from build123d import *

# Parameters (mm, degrees)
SKETCH1_R           = 17.5
SKETCH1_R_2         = 10
SKETCH1_R_3         = 2
BOSS_EXTRUDE1_DEPTH = 3.5
SKETCH3_R           = 10.5
BOSS_EXTRUDE2_DEPTH = 14
FILLET1_R           = 4
SKETCH4_R           = 6
BOSS_EXTRUDE3_DEPTH = 5
FILLET2_R           = 5


with BuildPart() as part:
    # Sketch1 → Boss-Extrude1 (new body)
    with BuildSketch(Plane.XY):
        Circle(SKETCH1_R)
        Circle(SKETCH1_R_2, mode=Mode.SUBTRACT)
        with Locations((6.70392983, 12.290538021)):
            Circle(SKETCH1_R_3, mode=Mode.SUBTRACT)
        with Locations((7.291953237, -11.951042548)):
            Circle(SKETCH1_R_3, mode=Mode.SUBTRACT)
        with Locations((-13.995883067, -0.339495473)):
            Circle(SKETCH1_R_3, mode=Mode.SUBTRACT)
    extrude(amount=BOSS_EXTRUDE1_DEPTH)

    # Sketch3 → Boss-Extrude2 (add)
    with BuildSketch(Plane.XY.offset(3.5)):
        Circle(SKETCH3_R)
    extrude(amount=BOSS_EXTRUDE2_DEPTH)

    # Fillet1
    fillet1_edges = [part.edges().sort_by_distance(p)[0] for p in [
        (-10.5, 0, 17.5),
    ]]
    fillet(fillet1_edges, radius=FILLET1_R)

    # Sketch4 → Boss-Extrude3 (add)
    with BuildSketch(Plane.XY.offset(17.5)):
        Circle(SKETCH4_R)
    extrude(amount=BOSS_EXTRUDE3_DEPTH)

    # Fillet2
    fillet2_edges = [part.edges().sort_by_distance(p)[0] for p in [
        (-6, 0, 22.5),
    ]]
    fillet(fillet2_edges, radius=FILLET2_R - 0.0001)  # a hair under: the kernel refuses the full size


solid = part.part
Work out the finished part from the listing and answer in its coordinate system (mm). A direction names the side the tool comes from. Coordinates: 2 decimals unless noted, no trailing zeros. Write each loop counter-clockwise with the first axis right and the second up, starting at its lowest first coordinate (ties: lowest second). Pieces come first, ordered by that corner, then holes.
1. The part is cut by section D-D, the plane x = 14. Write down the section's boundary in (y, z).
Results list:
outline: (-10.5, 0) - (10.5, 0) - (10.5, 3.5) - (-10.5, 3.5) - close
2. For faces 1 (the flat face through (0, 0, 3.5)), 2 (the flat face through (0, 0, 22.5)), 3 (the cylindrical face through (10, 3.2, 8.4)), determine the directions among +Z, -Z, +X, -X, +Y, -Y from which every point of the face is accessible in a straight line to the end or side of a thin tool.
Results list:
face 1: -Z
face 2: +Z, +X, -X, +Y, -Y
face 3: +Z
3. Consider line 1 along Y through (x, z) = (0, 0.8); line 2 along Y through (x, z) = (-14, 2); line 3 along Z through (x, y) = (-14.5, -8.5). Determine where each line is inside the solid, lowest interval first.
Results list:
line 1: y = -17.5 to -10, 10 to 17.5
line 2: y = -10.5 to -2.34, 1.66 to 10.5
line 3: z = 0 to 3.5
4. Flat-ended cylindrical pins translate along their axes: pin 1 (3 mm diameter, centred on x = -12.5, z = 12, fed in from +Y); pin 2 (1.5 mm diameter, centred on y = 7, z = 8, fed in from +X); pin 3 (12 mm diameter, centred on x = 7.5, z = 5, fed in from +Y); pin 4 (10.5 mm diameter, centred on x = 1, y = 4.5, fed in from +Z). Find the tip coordinate at first contact, or state that the pin passes through.
Results list:
pin 1: passes through
pin 2: stops at x = 8.44
pin 3: stops at y = 17.42
pin 4: stops at z = 22.5
5. The part is cut by section C-C, the plane z = 5.5. Write down the section's boundary in (x, y), and give its area (3 significant figures).
Results list:
outline: circle Ø21 at (0, 0)
area: 346 mm2
6. The part is cut by section B-B, the plane y = 11. Write down the section's boundary in (x, z).
Results list:
outline: (-13.61, 0) - (5.18, 0) - (5.18, 3.5) - (-13.61, 3.5) - close; (8.23, 0) - (13.61, 0) - (13.61, 3.5) - (8.23, 3.5) - close
7. The part is cut by section A-A, the plane x = -14. Write down the section's boundary in (y, z), and give its area (3 significant figures).
Results list:
outline: (-10.5, 0) - (-2.34, 0) - (-2.34, 3.5) - (-10.5, 3.5) - close; (1.66, 0) - (10.5, 0) - (10.5, 3.5) - (1.66, 3.5) - close
area: 59.5 mm2
